Here's how the part is built. I have some questions about the finished solid (model axes, mm). Face numbers are marked on the shaded views. A direction names the side the tool comes from. Give positions to 0.01 mm unless a question says otherwise; leave off trailing zeros. Order: outer loops, then holes, each group sorted by start corner. A loop starts at its lowest first (then second) coordinate and runs counter-clockwise, first axis right, second up. Notation, with made-up numbers: M 2.25,15 L 46.25,15 A28 cw 46.25,39 Z; hole C 21,19.5 d8. An arc over 180 degrees is marked long. Use one line per item in the form item = value.
from build123d import *

# Parameters (mm, degrees)
SKETCH2_W             = 10
SKETCH2_H             = 15
BOSS_EXTRUDE1_DEPTH   = 12
BOSS_EXTRUDE1_2_DEPTH = 12
BOSS_EXTRUDE2_DEPTH   = 30
CUT_EXTRUDE3_START    = -0.8
SKETCH5_W             = 26
SKETCH5_H             = 6.35
CUT_EXTRUDE3_DEPTH    = 13
SKETCH9_W             = 6.5
SKETCH9_H             = 6.5
CUT_EXTRUDE7_DEPTH    = 129.938939037
SKETCH11_W            = 11.4
SKETCH11_H            = 7.5
BOSS_EXTRUDE3_DEPTH   = 4
SKETCH12_W            = 10
SKETCH12_H            = 3
BOSS_EXTRUDE4_DEPTH   = 105
SKETCH13_W            = 6
SKETCH13_H            = 13
CUT_EXTRUDE9_DEPTH    = 129.938939037
SKETCH16_W            = 0.4
SKETCH16_H            = 6.35
BOSS_EXTRUDE5_DEPTH   = 0.15
CHAMFER3_SIZE         = 0.5


with BuildPart() as part:
    # Sketch2 → Boss-Extrude1 (new body)
    with BuildSketch(Plane(origin=(0, 0, 0), x_dir=(1, 0, 0), z_dir=(0, 1, 0))):
        Rectangle(SKETCH2_W, SKETCH2_H)
        Polygon((-1.75, -1.010362971), (0, -2.020725942), (1.75, -1.010362971), (1.75, 1.010362971), (0, 2.020725942), (-1.75, 1.010362971), align=None, mode=Mode.SUBTRACT)
    extrude(amount=BOSS_EXTRUDE1_DEPTH)


with BuildPart() as body_2:
    # Sketch2 → Boss-Extrude1 2 (new body)
    with BuildSketch(Plane(origin=(0, 0, 0), x_dir=(1, 0, 0), z_dir=(0, 1, 0))):
        with Locations((0, 120)):
            Rectangle(SKETCH2_W, SKETCH2_H)
        with BuildLine():
            Line((-2, 117.5), (-2, 122.5))
            ThreePointArc((-2, 122.5), (0, 124.5), (2, 122.5))
            Line((2, 122.5), (2, 117.5))
            ThreePointArc((2, 117.5), (0, 115.5), (-2, 117.5))
        make_face(mode=Mode.SUBTRACT)
    extrude(amount=BOSS_EXTRUDE1_2_DEPTH)



with BuildPart() as body_3:
    # Sketch3 → Boss-Extrude2 (new body)
    with BuildSketch(Plane.XY.offset(7.5)):
        Polygon((-1.4, 22.5), (1.1, 22.5), (1.1, 15), (12.5, 15), (12.5, 22.5), (15, 22.5), (15, 12), (-5, 12), (-5, 18.9), align=None)
    extrude(amount=-BOSS_EXTRUDE2_DEPTH)

    # Sketch5 → Cut-Extrude3 (cut)
    with BuildSketch(Plane.ZY.offset(-12.5).offset(CUT_EXTRUDE3_START)):
        with Locations((-9.5, 18.175)):
            Rectangle(SKETCH5_W, SKETCH5_H)
    extrude(amount=CUT_EXTRUDE3_DEPTH, mode=Mode.SUBTRACT)

    # Sketch9 → Cut-Extrude7 (cut, through all)
    with BuildSketch(Plane(origin=(0, 12, 0), x_dir=(1, 0, 0), z_dir=(0, 1, 0))):
        Rectangle(SKETCH9_W, SKETCH9_H)
    extrude(amount=CUT_EXTRUDE7_DEPTH, mode=Mode.SUBTRACT)

    # Sketch11 → Boss-Extrude3 (add)
    with BuildSketch(Plane.XY.offset(7.5)):
        with Locations((6.8, 18.75)):
            Rectangle(SKETCH11_W, SKETCH11_H)
    extrude(amount=-BOSS_EXTRUDE3_DEPTH)


with BuildPart() as body_2_1:
    add(body_2.part)

    add(body_3.part)  # Boss-Extrude4 merges body 3
    # Sketch12 → Boss-Extrude4 (add)
    with BuildSketch(Plane(origin=(0, 0, -22.5), x_dir=(-1, 0, 0), z_dir=(0, 0, -1))):
        with Locations((0, 13.5)):
            Rectangle(SKETCH12_W, SKETCH12_H)
    extrude(amount=BOSS_EXTRUDE4_DEPTH)

    # Sketch13 → Cut-Extrude9 (cut, through all)
    with BuildSketch(Plane.XZ.offset(-12)):
        with Locations((0, -120)):
            Rectangle(SKETCH13_W, SKETCH13_H)
    extrude(amount=-CUT_EXTRUDE9_DEPTH, mode=Mode.SUBTRACT)

    # Combine2: union part
    add(part.part)

    # Sketch16 → Boss-Extrude5 (add)
    with BuildSketch(Plane.ZY.offset(-13.3)):
        with Locations((-17.3, 18.175)):
            Rectangle(SKETCH16_W, SKETCH16_H)
        with Locations((-12.3, 18.175)):
            Rectangle(SKETCH16_W, SKETCH16_H)
        with Locations((-7.3, 18.175)):
            Rectangle(SKETCH16_W, SKETCH16_H)
        with Locations((-2.3, 18.175)):
            Rectangle(SKETCH16_W, SKETCH16_H)
    extrude(amount=BOSS_EXTRUDE5_DEPTH)

    # Chamfer3
    chamfer3_edges = [body_2_1.edges().sort_by_distance(p)[0] for p in [
        (10, 12, -22.5),
        (5, 7.5, -127.5),
        (5, 15, -75),
        (5, 13.5, -22.5),
        (0, 15, -127.5),
        (-5, 15, -75),
        (-2.35, 15, -22.5),
        (-5, 7.5, -127.5),
        (-5, 12, -60),
        (5, 12, -67.5),
        (0, 12, -112.5),
        (-2, 0, -120),
        (0, 0, -115.5),
        (2, 0, -120),
        (0, 0, -124.5),
        (5, 0, -120),
        (5, 6, -112.5),
        (0, 0, -127.5),
        (-5, 0, -120),
        (0, 0, -112.5),
        (-5, 6, -112.5),
        (15, 17.25, 7.5),
        (-5, 9.45, 7.5),
        (15, 17.25, -22.5),
        (10, 12, 7.5),
        (5, 12, 0),
        (0, 12, -7.5),
        (-0.875, 0, -1.515544457),
        (-1.75, 0, 0),
        (-0.875, 0, 1.515544457),
        (0.875, 0, 1.515544457),
        (1.75, 0, 0),
        (0.875, 0, -1.515544457),
        (5, 0, 0),
        (5, 6, 7.5),
        (0, 0, -7.5),
        (5, 6, -7.5),
        (-5, 0, 0),
        (-5, 6, -7.5),
        (0, 0, 7.5),
        (15, 12, -7.5),
        (13.75, 22.5, -22.5),
        (12.5, 21.925, -22.5),
        (9.15, 15, -22.5),
        (1.1, 21.925, -22.5),
        (12.9, 21.35, -22.5),
        (-0.15, 22.5, -22.5),
        (0.7, 21.35, -22.5),
        (0.3, 18.175, -22.5),
        (13.3, 18.175, -22.5),
        (-3.2, 20.7, -22.5),
        (-5, 16.95, -22.5),
        (0.3, 15, -12.875),
        (-3.2, 20.7, 7.5),
        (6.8, 22.5, 7.5),
    ]]
    chamfer(chamfer3_edges, length=CHAMFER3_SIZE)


solid = body_2_1.part
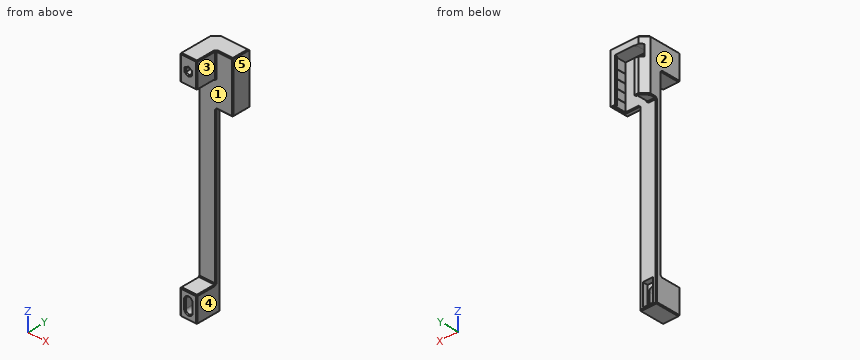
Q1. I want a section at A-A on y = 4.25. Write out the boundary of the cut face in (x, z), then the cut area to 3 significant figures.
Found:
outline = M -5,-127 L -4.5,-127.5 L 4.5,-127.5 L 5,-127 L 5,-113 L 4.5,-112.5 L -4.5,-112.5 L -5,-113 Z; M -5,-7 L -4.5,-7.5 L 4.5,-7.5 L 5,-7 L 5,7 L 4.5,7.5 L -4.5,7.5 L -5,7 Z; hole M -2,-122.5 A2 ccw 2,-122.5 L 2,-117.5 A2 ccw -2,-117.5 Z; hole M -1.75,-1.01 L 0,-2.02 L 1.75,-1.01 L 1.75,1.01 L 0,2.02 L -1.75,1.01 Z
area = 256 mm²
Q2. Thinking about a two-plate mould opening in Z: for the marked faces 1 and 2, which applies, +Z half, -Z half, draft (parallel to the pull), parting line (faces both ways), or undercut?
Found:
face_1 = undercut
face_2 = draft
Q3. I want a section at B-B on z = -71. Write out the boundary of the cut face in (x, y).
Found:
outline = M -5,12.5 L -4.5,12 L 4.5,12 L 5,12.5 L 5,14.5 L 4.5,15 L -4.5,15 L -5,14.5 Z
Q4. On a 3-axis mill with a long thin cutter (end or side, diameter ignored), from which of +Z, -Z, +X, -X, +Y, -Y can I reach the whole of each face in a straight line? I mean the marked faces 3, 4 and 5. Say none if no direction works.
Found:
face_3 = +Z, -Z, +X, -Y
face_4 = -Z, +X, +Y, -Y
face_5 = +Z, -Z, +X, +Y, -Y
Q5. I'm going to push flat-ended pins straight in: pin 1 Ø7 at (x, y) = (9.5, 17) entering from -Z; pin 2 Ø0.9 at (x, z) = (13, -11) entering from -Y; pin 3 Ø3 at (x, z) = (0.5, -97.5) entering from +Y; pin 4 Ø6 at (x, z) = (9.5, -30.5) entering from +Y. Where does each tip first touch, or does it pass through?
Found:
pin_1 = -22.5
pin_2 = 12
pin_3 = 15
pin_4 = through
Q6. I need wall thicknesses on L1, parallel to Z at x = 0.25, y = 12.25; L2, parallel to Z at x = -2.25, y = 7.5; L3, parallel to Z at x = -0.5, y = 2.75. Which ranges of each line are inside material? Lowest first, please.
Found:
L1 = -127.5 to -126.5, -113.5 to -3.25, 3.25 to 7.5
L2 = -127.5 to -112.5, -7.5 to 7.5
L3 = -127.5 to -124.44, -115.56 to -112.5, -7.5 to -1.73, 1.73 to 7.5
